Here's how the part is built. I have some questions about the finished solid (model axes, mm). Round coordinates to 2 decimals unless told otherwise and drop trailing zeros. Write each loop counter-clockwise with the first axis right and the second up, starting at its lowest first coordinate (ties: lowest second). Pieces come first, ordered by that corner, then holes. Notation, with made-up numbers: M 89,89.5 L 129,89.5 A33 ccw 129,120.5 Z; hole C 58.5,74 d10. An arc over 180 degrees is marked long. Write item = value, one per line. Start each with the question number.
(1) Will this pin go through, and if not, where does the flat tip stop? pin 1 Ø3 at (x, y) = (38, 1) entering from +Z.
(2) I want a section at B-B (x = 14.5). List the corners of the cut face in (y, z) for me, and give its area (3 significant figures).
(3) I want a section at C-C (z = -9). List the corners of the cut face in (x, y) for me, and give its area (3 significant figures).
(4) I want a section at D-D (z = 0). List the corners of the cut face in (x, y) for me.
(5) I need wall thicknesses on line 1 along Z through (x, y) = (43.5, 0); line 2 along Z through (x, y) = (47.5, 6); line 3 along Y through (x, z) = (22, 8.75). Which ranges of each line are inside material? Lowest first, please.
(6) If we mould it in two halves opening along X, with no side actions, what happens to faces 1 (the cylindrical face through (32.8, -2.4, 7.8)), 2 (the flat face through (0, -5.4, 0.2)), 3 (the flat face through (72, -5.4, 0.2)), 4 (the flat face through (35, -12.5, 0))? For each: released by +X, released by -X, zero draft, split by the parting line, or undercut.
(7) I want a section at A-A (y = 0). List the corners of the cut face in (x, z) for me.
```python
from build123d import *

# Parameters (mm, degrees)
SKETCH1_W           = 25
SKETCH1_H           = 25
SKETCH1_R           = 5
BOSS_EXTRUDE1_DEPTH = 72
SKETCH2_R           = 4
CUT_EXTRUDE1_DEPTH  = 78.235030912


with BuildPart() as part:
    # Sketch1 → Boss-Extrude1 (new body)
    with BuildSketch(Plane(origin=(0, 0, 0), x_dir=(0, 0, -1), z_dir=(1, 0, 0))):
        Rectangle(SKETCH1_W, SKETCH1_H)
        Circle(SKETCH1_R, mode=Mode.SUBTRACT)
        with BuildLine():
            Line((-11.5, -11.5), (-3.4278273, -11.5))
            ThreePointArc((-3.4278273, -11.5), (-8.485281374, -8.485281374), (-11.5, -3.4278273))
            Line((-11.5, -3.4278273), (-11.5, -11.5))
        make_face(mode=Mode.SUBTRACT)
        with BuildLine():
            Line((-11.5, 11.5), (-3.4278273, 11.5))
            ThreePointArc((-3.4278273, 11.5), (-8.485281374, 8.485281374), (-11.5, 3.4278273))
            Line((-11.5, 3.4278273), (-11.5, 11.5))
        make_face(mode=Mode.SUBTRACT)
        with BuildLine():
            Line((11.5, -11.5), (11.5, -3.4278273))
            ThreePointArc((11.5, -3.4278273), (8.485281374, -8.485281374), (3.4278273, -11.5))
            Line((3.4278273, -11.5), (11.5, -11.5))
        make_face(mode=Mode.SUBTRACT)
        with BuildLine():
            Line((3.4278273, 11.5), (11.5, 11.5))
            Line((11.5, 11.5), (11.5, 3.4278273))
            ThreePointArc((11.5, 3.4278273), (8.485281374, 8.485281374), (3.4278273, 11.5))
        make_face(mode=Mode.SUBTRACT)
    extrude(amount=BOSS_EXTRUDE1_DEPTH)

    # Sketch2 → Cut-Extrude1 (cut, through all)
    with BuildSketch(Plane.XY.offset(12.5)):
        with Locations((36, 0)):
            Circle(SKETCH2_R)
    extrude(amount=-CUT_EXTRUDE1_DEPTH, mode=Mode.SUBTRACT)


solid = part.part
```
Returned:
q1.pin_1 = through
q2.outline = M -12.5,-12.5 L 12.5,-12.5 L 12.5,12.5 L -12.5,12.5 Z; hole M -11.5,-11.5 L -3.43,-11.5 A12 cw -11.5,-3.43 Z; hole M -11.5,3.43 A12 cw -3.43,11.5 L -11.5,11.5 Z; hole C 0,0 d10; hole M 3.43,-11.5 L 11.5,-11.5 L 11.5,-3.43 A12 cw Z; hole M 3.43,11.5 A12 cw 11.5,3.43 L 11.5,11.5 Z
q2.area = 461 mm²
q3.outline = M 0,-12.5 L 72,-12.5 L 72,-11.5 L 0,-11.5 Z; M 0,-7.94 L 72,-7.94 L 72,7.94 L 0,7.94 Z; M 0,11.5 L 72,11.5 L 72,12.5 L 0,12.5 Z; hole C 36,0 d8
q3.area = 1,240 mm²
q4.outline = M 0,-12.5 L 72,-12.5 L 72,-5 L 0,-5 Z; M 0,5 L 72,5 L 72,12.5 L 0,12.5 Z
q5.line_1 = -12.5 to -5, 5 to 12.5
q5.line_2 = -12.5 to -11.5, -10.39 to 10.39, 11.5 to 12.5
q5.line_3 = -12.5 to -11.5, -8.21 to 8.21, 11.5 to 12.5
q6.face_1 = undercut
q6.face_2 = released by -X
q6.face_3 = released by +X
q6.face_4 = zero draft
q7.outline = M 0,-12.5 L 32,-12.5 L 32,-5 L 0,-5 Z; M 0,5 L 32,5 L 32,12.5 L 0,12.5 Z; M 40,-12.5 L 72,-12.5 L 72,-5 L 40,-5 Z; M 40,5 L 72,5 L 72,12.5 L 40,12.5 Z
